Geometry check sheet. Reference: drawing and pictorial views, mm from the part's lowest x, y, z. Give positions to 0.01 mm unless a question says otherwise; leave off trailing zeros. Loops run counter-clockwise (first coordinate to the right, second up) from the corner with the lowest first, then second, coordinate; pieces in that order, holes last. Notation, with made-up numbers: M 15.5,12 L 25.5,12 A28 ccw 25.5,32 Z; hole C 89.5,-32.5 d11. An arc over 180 degrees is marked long. Put each result on its own line as item: value. Start each with the question number.
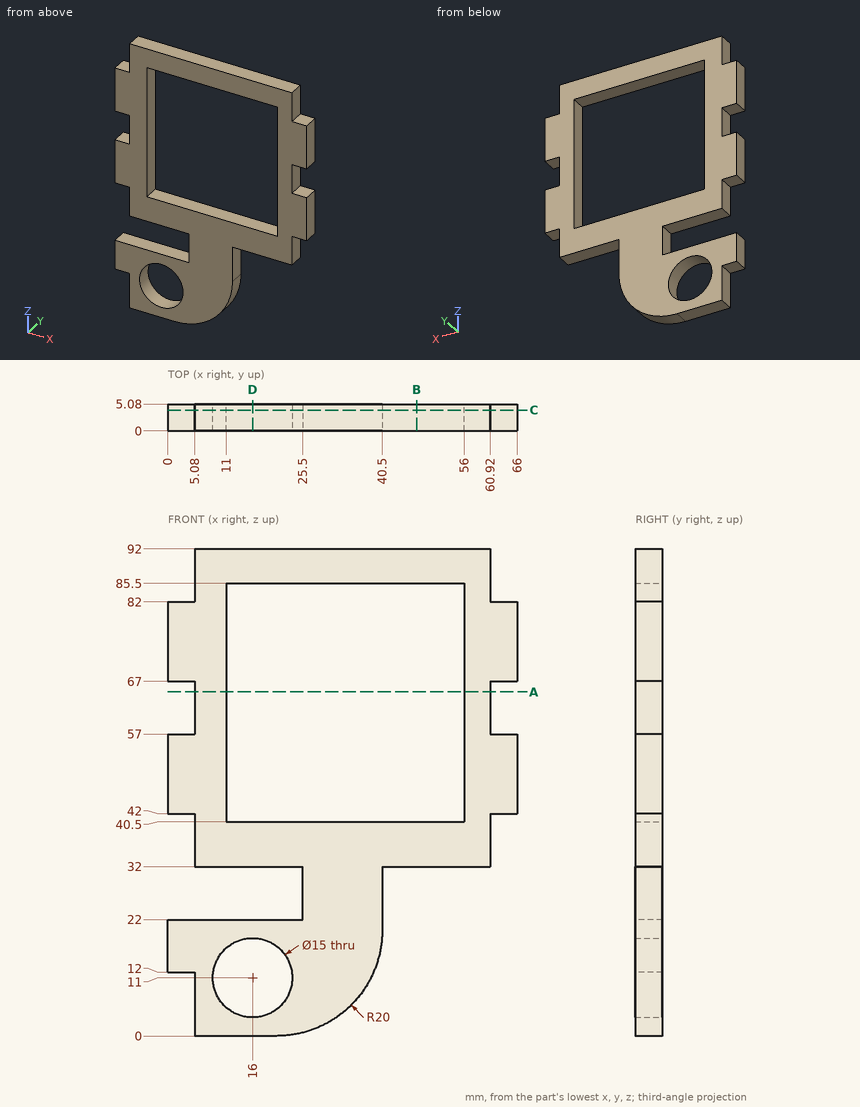
Q1. Depth check by flat-ended pin: P1, Ø1.5, axis at x = 64, y = 3, coming from the +Z side; P2, Ø2.5, axis at x = 3, y = 3, coming from the -Z side; P3, Ø2.5, axis at y = 2, z = 89.5, coming from the -X side. Enter the tip coordinate at first touch or a pass-through.
Q2. Section check B-B, the plane x = 47. Record the cut outline in (y, z), then the cut area to 3 significant figures.
Q3. Section check A-A, the plane z = 65. Record the cut outline in (x, y), then the cut area to 3 significant figures.
Q4. Section check C-C, the plane y = 3.9. Give the number of separate pieces and of enclosed holes in the cut face, then the cut area to 3 significant figures.
Q5. Section check D-D, the plane x = 16. Record the cut outline in (y, z), then the cut area to 3 significant figures.
Q6. Thickness scan on line 1 along Z through (x, y) = (16, 1.25); line 2 along X through (y, z) = (0.45, 79.5); line 3 along Z through (x, y) = (53, 2.75). Record the ranges inside material, lowest first. Write a range as [from, to].
Found:
1. P1: stops at z = 82
1. P2: stops at z = 12
1. P3: stops at x = 5.08
2. outline: M 0,32 L 5.08,32 L 5.08,40.5 L 0,40.5 Z; M 0,85.5 L 5.08,85.5 L 5.08,92 L 0,92 Z
2. area: 76.2 mm^2
3. outline: M 5.08,0 L 11,0 L 11,5.08 L 5.08,5.08 Z; M 56,0 L 60.92,0 L 60.92,5.08 L 56,5.08 Z
3. area: 55.1 mm^2
4. separate pieces: 1
4. enclosed holes: 2
4. area: 2,350 mm^2
5. outline: M 0,0 L 5.08,0 L 5.08,3.5 L 0,3.5 Z; M 0,18.5 L 5.08,18.5 L 5.08,22 L 0,22 Z; M 0,32 L 5.08,32 L 5.08,40.5 L 0,40.5 Z; M 0,85.5 L 5.08,85.5 L 5.08,92 L 0,92 Z
5. area: 112 mm^2
6. line 1: z = [0, 3.5], [18.5, 22], [32, 40.5], [85.5, 92]
6. line 2: x = [0, 11], [56, 66]
6. line 3: z = [32, 40.5], [85.5, 92]
